Drawing for the job (mm, zero at the part's lowest x, y, z). A direction names the side the tool comes from. Round coordinates to 2 decimals unless told otherwise and drop trailing zeros. Loops run counter-clockwise (first coordinate to the right, second up) from the corner with the lowest first, then second, coordinate; pieces in that order, holes last. Notation, with made-up numbers: (52, 2) - (74, 2) arc R29 cw to (74, 22) - close; hole circle Ø2 at (84, 70). An arc over 180 degrees is marked (long way). Put each result on its own line as item: value.
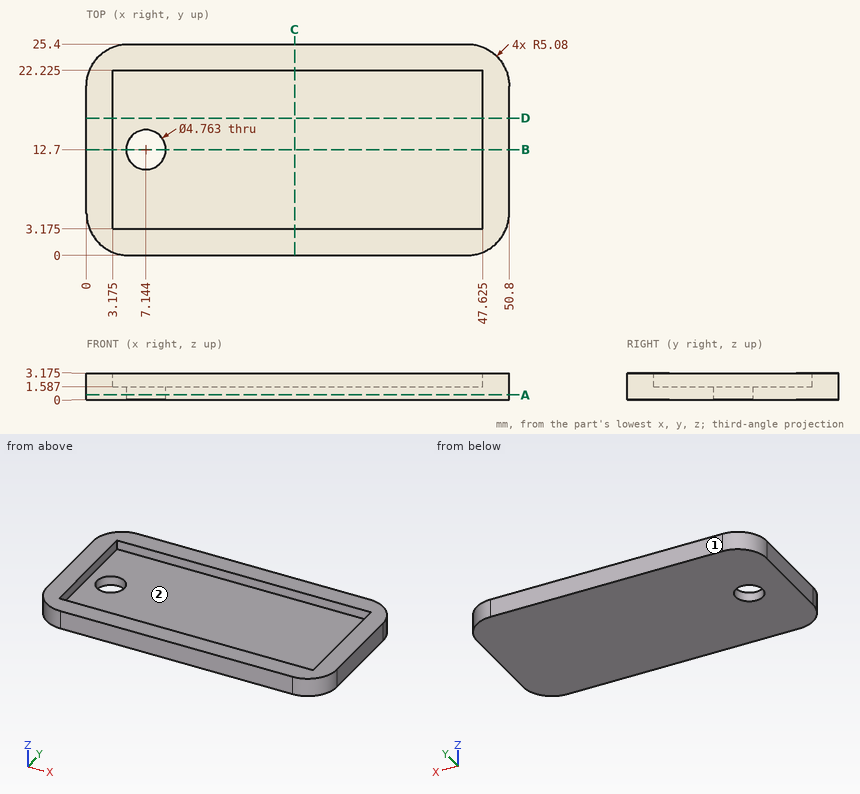
1. Band-saw the part on D-D (y = 16.5). List the corners of the cut face in (x, z) (1 decimal).
A:
outline: (0, 0) - (50.8, 0) - (50.8, 3.2) - (47.6, 3.2) - (47.6, 1.6) - (3.2, 1.6) - (3.2, 3.2) - (0, 3.2) - close
2. Pin check, flat tips, straight feed: P1, Ø1.3, axis at y = 14, z = 2.5, coming from the -X side; P2, Ø5.5, axis at x = 20.5, y = 17, coming from the +Z side. Stop position of each tip, or through.
A:
P1: stops at x = 0
P2: stops at z = 1.59
3. Band-saw the part on C-C (x = 25). List the corners of the cut face in (y, z) (1 decimal).
A:
outline: (0, 0) - (25.4, 0) - (25.4, 3.2) - (22.2, 3.2) - (22.2, 1.6) - (3.2, 1.6) - (3.2, 3.2) - (0, 3.2) - close
4. Band-saw the part on A-A (z = 0.6). List the corners of the cut face in (x, y) (1 decimal), plus the area to 3 significant figures.
A:
outline: (0, 5.1) arc R5.1 ccw to (5.1, 0) - (45.7, 0) arc R5.1 ccw to (50.8, 5.1) - (50.8, 20.3) arc R5.1 ccw to (45.7, 25.4) - (5.1, 25.4) arc R5.1 ccw to (0, 20.3) - close; hole circle Ø4.8 at (7.1, 12.7)
area: 1,250 mm²
5. Band-saw the part on B-B (y = 12.7). List the corners of the cut face in (x, z) (1 decimal).
A:
outline: (0, 0) - (4.8, 0) - (4.8, 1.6) - (3.2, 1.6) - (3.2, 3.2) - (0, 3.2) - close; (9.5, 0) - (50.8, 0) - (50.8, 3.2) - (47.6, 3.2) - (47.6, 1.6) - (9.5, 1.6) - close
6. Probe line 1 along X through (y, z) = (15.25, 2.2) (1 decimal); line 2 along Y through (x, z) = (18.5, 2.4) (1 decimal); line 3 along X through (y, z) = (13, 1.1) (1 decimal). List the from-to ranges inside material, lowest first. Write a range as [from, to].
A:
line 1: x = [0, 3.2], [47.6, 50.8]
line 2: y = [0, 3.2], [22.2, 25.4]
line 3: x = [0, 4.8], [9.5, 50.8]
7. Tool access for the marked faces 1 and 2: list every direction of +Z, -Z, +X, -X, +Y, -Y with a clear straight run to the whole face (end or side of a thin tool).
A:
face 1: +Z, -Z, +X, -X, +Y
face 2: +Z
